```python
from build123d import *

# Parameters (mm, degrees)
SKETCH1_R           = 2.2225
BOSS_EXTRUDE2_DEPTH = 7.62
CUT_EXTRUDE1_DEPTH  = 6.35
CUT_EXTRUDE7_DEPTH  = 6.35
CUT_EXTRUDE8_DEPTH  = 6.35
SKETCH5_W           = 8.89
SKETCH5_H           = 15.494
SKETCH5_R           = 2.2225
BOSS_EXTRUDE3_DEPTH = 7.62


with BuildPart() as part:
    # Sketch1 → Boss-Extrude2 (new body)
    with BuildSketch(Plane(origin=(0, 0, 0), x_dir=(1, 0, 0), z_dir=(0, 1, 0))):
        Polygon((3.666174209, 11.65), (-3.666174209, 11.65), (-11.922283059, -2.65), (-8.256108849, -9), (8.256108849, -9), (11.922283059, -2.65), align=None)
        with Locations(Location((0, 0, 0), (0, 0, 90))):
            Circle(SKETCH1_R, mode=Mode.SUBTRACT)
    extrude(amount=BOSS_EXTRUDE2_DEPTH)

    # Sketch2 → Cut-Extrude1 (cut)
    with BuildSketch(Plane(origin=(-10.089195954, 0, 5.825), x_dir=(0.5000000000000006, 0, 0.8660254037844384), z_dir=(-0.8660254037844384, 0, 0.5000000000000006))):
        with BuildLine():
            ThreePointArc((0, 1.81), (1.414213562, 2.395786438), (2, 3.81))
            Line((2, 3.81), (0, 3.81))
            Line((0, 3.81), (0, 1.81))
        make_face()
        with BuildLine():
            Line((0, 3.81), (2, 3.81))
            ThreePointArc((2, 3.81), (1.414213562, 5.224213562), (0, 5.81))
            Line((0, 5.81), (0, 3.81))
        make_face()
        with BuildLine():
            Line((0, 1.81), (0, 3.81))
            Line((0, 3.81), (-2, 3.81))
            ThreePointArc((-2, 3.81), (-1.414213562, 2.395786438), (0, 1.81))
        make_face()
        with BuildLine():
            Line((-2, 3.81), (0, 3.81))
            Line((0, 3.81), (0, 5.81))
            ThreePointArc((0, 5.81), (-1.414213562, 5.224213562), (-2, 3.81))
        make_face()
    extrude(amount=-CUT_EXTRUDE1_DEPTH, mode=Mode.SUBTRACT)

    # Sketch3 → Cut-Extrude7 (cut)
    with BuildSketch(Plane(origin=(10.089195954, 0, 5.825), x_dir=(0.49999999999999983, 0, -0.8660254037844388), z_dir=(0.8660254037844387, 0, 0.4999999999999998))):
        with BuildLine():
            ThreePointArc((2, 3.81), (1.414213562, 5.224213562), (0, 5.81))
            Line((0, 5.81), (0, 3.81))
            Line((0, 3.81), (2, 3.81))
        make_face()
        with BuildLine():
            Line((0, 3.81), (0, 5.81))
            ThreePointArc((0, 5.81), (-1.414213562, 5.224213562), (-2, 3.81))
            Line((-2, 3.81), (0, 3.81))
        make_face()
        with BuildLine():
            Line((2, 3.81), (0, 3.81))
            Line((0, 3.81), (0, 1.81))
            ThreePointArc((0, 1.81), (1.414213562, 2.395786438), (2, 3.81))
        make_face()
        with BuildLine():
            Line((0, 1.81), (0, 3.81))
            Line((0, 3.81), (-2, 3.81))
            ThreePointArc((-2, 3.81), (-1.414213562, 2.395786438), (0, 1.81))
        make_face()
    extrude(amount=-CUT_EXTRUDE7_DEPTH, mode=Mode.SUBTRACT)

    # Sketch4 → Cut-Extrude8 (cut)
    with BuildSketch(Plane(origin=(0, 0, -11.65), x_dir=(-1, 0, 0), z_dir=(0, 0, -1))):
        with BuildLine():
            ThreePointArc((2, 3.81), (1.414213562, 5.224213562), (0, 5.81))
            Line((0, 5.81), (0, 3.81))
            Line((0, 3.81), (2, 3.81))
        make_face()
        with BuildLine():
            Line((0, 3.81), (0, 5.81))
            ThreePointArc((0, 5.81), (-1.414213562, 5.224213562), (-2, 3.81))
            Line((-2, 3.81), (0, 3.81))
        make_face()
        with BuildLine():
            Line((2, 3.81), (0, 3.81))
            Line((0, 3.81), (0, 1.81))
            ThreePointArc((0, 1.81), (1.414213562, 2.395786438), (2, 3.81))
        make_face()
        with BuildLine():
            Line((0, 1.81), (0, 3.81))
            Line((0, 3.81), (-2, 3.81))
            ThreePointArc((-2, 3.81), (-1.414213562, 2.395786438), (0, 1.81))
        make_face()
    extrude(amount=-CUT_EXTRUDE8_DEPTH, mode=Mode.SUBTRACT)

    # Sketch5 → Boss-Extrude3 (add)
    # profile 1 of 3: a face of its own
    with BuildSketch(Plane.XZ):
        with Locations((0, 16.747)):
            Rectangle(SKETCH5_W, SKETCH5_H)
        with Locations(Location((0, 20.09, 0), (0, 0, 270))):
            Circle(SKETCH5_R, mode=Mode.SUBTRACT)
    # profile 2 of 3: a face of its own
    with BuildSketch(Plane.XZ):
        Polygon((-5.571728634, -8.34948292), (-10.016728634, -0.65051708), (-23.43492624, -8.39751708), (-18.98992624, -16.09648292), align=None)
        with Locations(Location((-17.398450362, -10.045, 0), (0, 0, 270))):
            Circle(SKETCH5_R, mode=Mode.SUBTRACT)
    # profile 3 of 3: a face of its own
    with BuildSketch(Plane.XZ):
        Polygon((10.016728634, -0.65051708), (5.571728634, -8.34948292), (18.98992624, -16.09648292), (23.43492624, -8.39751708), align=None)
        with Locations(Location((17.398450362, -10.045, 0), (0, 0, 270))):
            Circle(SKETCH5_R, mode=Mode.SUBTRACT)
    extrude(amount=-BOSS_EXTRUDE3_DEPTH)


solid = part.part
```
Input: part model. Units: mm. Frame: model coordinates. A direction names the side the tool comes from. Round coordinates to 2 decimals unless told otherwise and drop trailing zeros. Loops run counter-clockwise (first coordinate to the right, second up) from the corner with the lowest first, then second, coordinate; pieces in that order, holes last. Notation, with made-up numbers: M 7.25,41.25 L 21.25,41.25 A30 ccw 21.25,73.25 Z; hole C 45,60 d5. An arc over 180 degrees is marked long. Answer in a Markdown table with one row per item. Add a question column.
1. Section C-C (z = -6). Output: boundary loops of the cut face in (x, y), and give its area (3 significant figures).
2. Section D-D (z = 16). Output: boundary loops of the cut face in (x, y) (3 decimals).
3. Ray query, probe 1 along X at (y, z) = (4, 1.5); probe 2 along X at (y, z) = (7.25, -8.5); probe 3 along Z at (x, y) = (-2, 0.5). Return the intervals inside material, ascending.
4. Set-up query: faces 4 (the face through (-2, 2, -11.65)), 5 (the face through (6, 4, 9)), 6 (the face through (-6, 4, 9)). Return all of +Z, -Z, +X, -X, +Y, -Y with unobstructed straight access to the full face (end or side cutting, diameter ignored); none if empty.
5. Section A-A (z = 20.09). Output: boundary loops of the cut face in (x, y) (1 decimal).
6. Contact query for flat-ended pins moving along their axis: pin 1 (10 mm diameter, centred on x = 9, z = 9.5, fed in from +Y); pin 2 (4 mm diameter, centred on x = 6.5, y = 2, fed in from +Z); pin 3 (4 mm diameter, centred on y = 5, z = -0.5, fed in from -X); pin 4 (1.2 mm diameter, centred on x = -0.5, y = 4.5, fed in from -Z). Output: stop coordinate, or through.
7. Mould query, pull axis Z, two halves, no side actions, for faces 1 (the face through (-4.606, 3.757, -10.023)), 2 (the face through (-4.445, 4, 17)), 3 (the face through (2.17, 3.76, 0.48)). Classes: released by +Z, released by -Z, zero draft, split by the parting line, or undercut.
8. Section B-B (x = -18). Output: boundary loops of the cut face in (y, z).
Values follow:
| question | item | result |
|---|---|---|
| 1 | outline | M -19.28,0 L 19.28,0 L 19.28,7.62 L -19.28,7.62 Z; hole C 0,3.81 d4 |
| 1 | area | 281 mm^2 |
| 2 | outline | M -4.445,0 L 4.445,0 L 4.445,7.62 L -4.445,7.62 Z |
| 3 | probe 1 | -11.26 to -6.58, -5.25 to -1.64, 1.64 to 5.25, 6.58 to 11.26 |
| 3 | probe 2 | -23.38 to -19, -15.8 to -5.83, -5.48 to 5.48, 5.83 to 15.8, 19 to 23.38 |
| 3 | probe 3 | -11.65 to -0.97, 0.97 to 19.12, 21.06 to 24.49 |
| 4 | face 4 | -Z, +Y, -Y |
| 4 | face 5 | +Z, +X, +Y, -Y |
| 4 | face 6 | +Z, -X, +Y, -Y |
| 5 | outline | M -4.4,0 L -2.2,0 L -2.2,7.6 L -4.4,7.6 Z; M 2.2,0 L 4.4,0 L 4.4,7.6 L 2.2,7.6 Z |
| 6 | pin 1 | y = 7.62 |
| 6 | pin 2 | z = 9 |
| 6 | pin 3 | x = -13.22 |
| 6 | pin 4 | z = -5.3 |
| 7 | face 1 | released by -Z |
| 7 | face 2 | zero draft |
| 7 | face 3 | undercut |
| 8 | outline | M 0,-15.52 L 7.62,-15.52 L 7.62,-12.18 L 0,-12.18 Z; M 0,-7.91 L 7.62,-7.91 L 7.62,-5.26 L 0,-5.26 Z |
